Autodesk Inventor part; units mm, degrees
ref_plane "YZ Plane" through (0, 0, 0) normal (1, 0, 0) x (0, 1, 0)
ref_plane "XZ Plane" through (0, 0, 0) normal (0, 1, 0) x (-1, 0, 0)
ref_plane "XY Plane" through (0, 0, 0) normal (0, 0, 1) x (1, 0, 0)
ref_plane "Work Plane1" through (0, 0, 0) normal (0, 0, 1) x (1, 0, 0)
sketch "Sketch1" plane through (0, 0, 0) normal (0, 0, 1) x (1, 0, 0)
  circle A0 centre (18.3844, -18.3844) radius 1.4
  circle A1 centre (-18.3822, 18.3822) radius 1.4
  arc A2 (9.6814, 2.5019) -> (1.0662, 9.9409) centre (9.4999, 11) ccw
  arc A3 (1.0662, 9.9409) -> (9.6814, 2.5019) centre (0, -0.0021) ccw
  circle A4 centre (0, 0) radius 30
ref_plane "Work Plane3" through (18.3844, -18.3844, 0) normal (0.7071, 0.7071, 0) x (-0.7071, 0.7071, 0)
ref_plane "Work Plane2" through (0, 0, 0) normal (0, 0, 1) x (1, 0, 0)
sketch "Sketch2" plane through (18.3844, -18.3844, 0) normal (0.7071, 0.7071, 0) x (-0.7071, 0.7071, 0)
  line L0 (55.9994, 0) -> (-4.0006, 0)
  line L1 (-4.0006, 0) -> (13.2067, 24.5746)
  line L2 (-4.0006, 0) -> (25.9994, 0) construction
  line L3 (22.8954, 10) -> (30.4529, 10)
  line L4 (-36.9123, 0) -> (106.4847, 0)
  line L5 (55.9994, 0) -> (38.7921, 24.5746)
  line L6 (55.9994, 0) -> (85.9994, 0) construction
  line L7 (38.7921, 24.5746) -> (13.2067, 24.5746)
  line L8 (0.8825, 0) -> (15.289, 20.5746)
  line L9 (15.289, 20.5746) -> (36.7098, 20.5746)
  line L10 (36.7098, 20.5746) -> (51.1163, 0)
  line L11 (55.9994, 0) -> (51.1163, 0)
  line L12 (0.8825, 0) -> (-4.0006, 0)
  point P0 (25.9994, 0)
  point P1 (0.8825, 0)
  point P2 (51.1163, 0)
  dimension "d1" = 30
  dimension "d2" = 55
  dimension "d3" = 125
  dimension "d5" = 4
  dimension "d6" = 4
  dimension "d7" = 4
extrude "Extrusion1" add sketch "Sketch2" along normal mid plane 20 contours L0 L10 L9 L8 L1 L7 L5
sketch "Sketch3" plane through (16.1169, -1.9747, 24.5746) normal (0, 0, 1) x (0.7071, 0.7071, 0)
  circle A0 centre (-10, 38.7891) radius 1.4
  circle A1 centre (-10, -13.2067) radius 1.4
  point P0 (-10, 12.7927)
hole "Hole1" at (-18.3822, 18.3822, 24.5746) at (18.3844, -18.3844, 24.5746) direction (0, 0, -1) diameter 2.8 end through all counterbore diameter 6.5 counterbore depth 22
sketch "Sketch4" plane through (16.1169, -1.9747, 24.5746) normal (0, 0, 1) x (0.7071, 0.7071, 0)
  circle A0 centre (-10.0015, 21.2913) radius 1.9
  line L0 (0, 0) -> (-20, 0)
  line L1 (0, 25.5854) -> (0, 0)
  line L2 (-20, 25.5854) -> (0, 25.5854)
  line L3 (-20, 0) -> (-20, 25.5854)
  circle A1 centre (-10.0015, 4.2912) radius 1.9
  circle A2 centre (-10.0015, 12.7912) radius 3
  circle A3 centre (-10.0015, 21.2913) radius 1.4
  circle A4 centre (-10.0015, 4.2912) radius 1.9
  circle A5 centre (-10.0015, 4.2912) radius 1.4
  point P0 (-10, 12.7927)
  dimension "d17" = 2.8
  dimension "d18" = 2.8
extrude "Extrusion2" cut sketch "Sketch4" against normal blind 20 contours A2 | A3 | A5
properties part number "Anglerfish_Lightplate_Tislinkbridge"
Verification items for the finished model (mm, model axes). A direction names the side the tool comes from. Coordinates: 2 decimals unless noted, no trailing zeros. Order: outer loops, then holes, each group sorted by start corner. A loop starts at its lowest first (then second) coordinate and runs counter-clockwise, first axis right, second up. Notation, with made-up numbers: M 56.5,13 L 106.5,13 A24 ccw 106.5,46 Z; hole C -27,9 d10. An arc over 180 degrees is marked long. One line per item, written item: value. Start each with the question number.
Item 1: Sectioned sample at A-A on z = 11.5. Record the cut outline in (x, y).
Item 2: Sectioned sample at B-B on y = 5.5. Record the cut outline in (x, z).
Item 3: Access from +Z, -Z, +X, -X, +Y, -Y to the whole of each face (thin tool, end or side, straight path). Record for faces 4 (the flat face through (16.9, -17.6, 2.575)), 5 (the flat face through (-3.2, -0.1, 20.575)), 6 (the flat face through (19, -20, 0)).
Item 4: Mould release check, pull along X, two halves, no side actions. Record for faces 1 (the flat face through (-4, 0, 24.575)), 2 (the cylindrical face through (1.611, -2.533, 22.603)), 3 (the flat face through (-12.69, 12.5, 10.43)): pulls with the +X half, pulls with the -X half, needs draft (parallel to the pull), parting line crosses it, or undercut.
Item 5: Sectioned sample at C-C on y = 13. Record the cut outline in (x, z), then the cut area to 3 significant figures.
Item 6: Sectioned sample at D-D on z = 21.25. Record the cut outline in (x, y).
Item 7: Thickness scan on probe 1 along X at (y, z) = (6, 12.5); probe 2 along Z at (x, y) = (-13.5, 19.5); probe 3 along Y at (x, z) = (8.5, 12). Record the ranges inside material, lowest first.
Item 8: Depth check by flat-ended pin: P1, Ø5.5, axis at x = 0, y = 0, coming from the +Z side; P2, Ø8, axis at x = 21.5, z = 21.5, coming from the -Y side; P3, Ø12, axis at x = 22, z = 21.5, coming from the -Y side; P4, Ø10, axis at y = 21, z = 14, coming from the -X side. Enter the tip coordinate at first touch or a pass-through.
Calculated:
1. outline: M -22.59,8.45 L -19.14,5 L -5,19.14 L -8.45,22.59 Z; M 5,-19.14 L 8.45,-22.59 L 22.59,-8.45 L 19.14,-5 Z
2. outline: M -19.64,10.48 L -9.65,20.57 L -7.31,20.57 L -7.31,24.57 L -12.59,24.57 L -19.64,17.45 Z; M -4.71,20.57 L 8.64,20.57 L 8.64,24.57 L -4.71,24.57 Z
3. face 4: +Z
3. face 5: -Z
3. face 6: -Z, +X, -X, +Y, -Y
4. face 1: needs draft
4. face 2: undercut
4. face 3: pulls with the +X half
5. outline: M -27.14,0 L -22.52,0 L -2.15,20.57 L 1.14,20.57 L 1.14,24.57 L -5.09,24.57 L -27.14,2.31 Z
5. area: 172 mm^2
6. outline: M -17.76,3.62 L 3.62,-17.76 L 17.76,-3.62 L -3.62,17.76 Z; hole C -6.01,6.01 d2.8; hole C -0.01,-0.01 d6.02; hole C 6.01,-6.01 d2.8
7. probe 1: -20.14 to -17.14
7. probe 2: 2.55 to 9.52
7. probe 3: -22.04 to -15.14
8. P1: through
8. P2: y = -5.27
8. P3: y = -7.58
8. P4: x = -14.6
